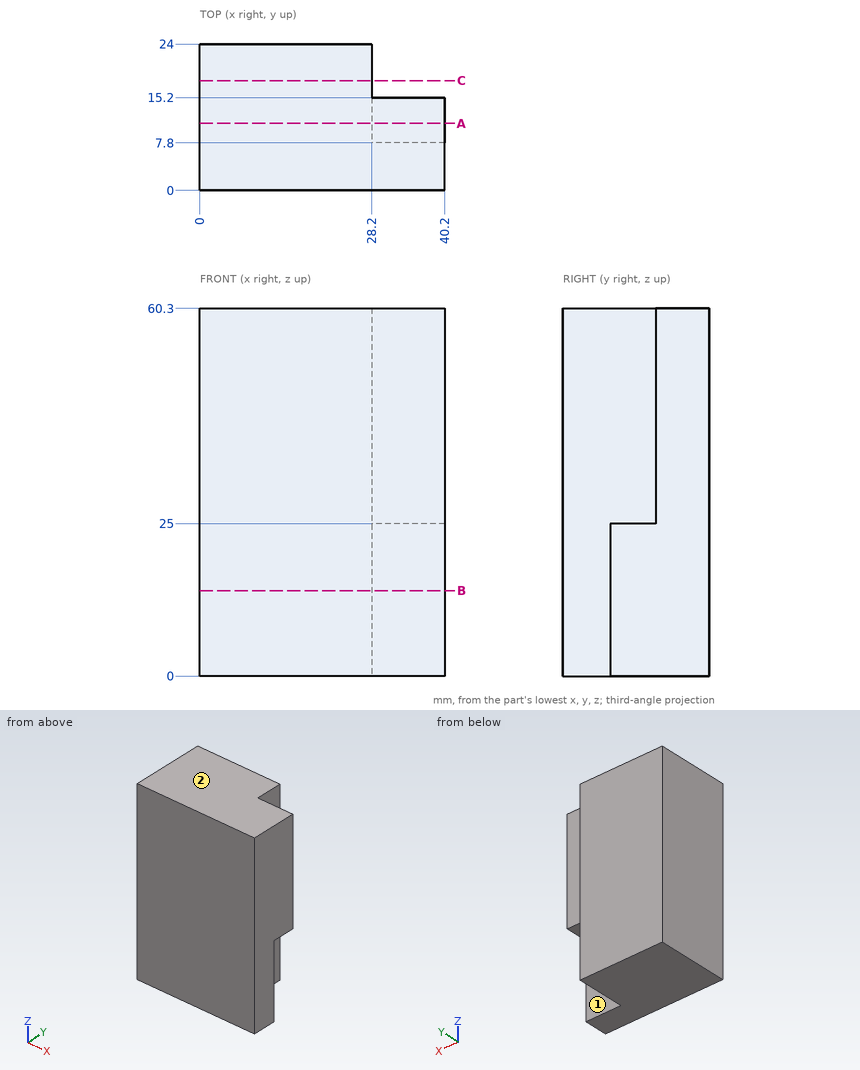
Drawing for the job (mm, zero at the part's lowest x, y, z). A direction names the side the tool comes from. Round coordinates to 2 decimals unless told otherwise and drop trailing zeros. Write each loop counter-clockwise with the first axis right and the second up, starting at its lowest first coordinate (ties: lowest second). Pieces come first, ordered by that corner, then holes.
Item 1: Band-saw the part on C-C on y = 18. Write the cut outline in (x, z).
Filled in:
outline: (0, 0) - (28.2, 0) - (28.2, 60.3) - (0, 60.3) - close
Item 2: Band-saw the part on A-A on y = 11. Write the cut outline in (x, z).
Filled in:
outline: (0, 0) - (28.2, 0) - (28.2, 25) - (40.2, 25) - (40.2, 60.3) - (0, 60.3) - close
Item 3: Drop flat-ended pins along their axis: pin 1 Ø2 at (x, y) = (34.5, 12.5) entering from -Z; pin 2 Ø2 at (y, z) = (18.5, 24.5) entering from +X; pin 3 Ø13 at (x, z) = (36, 14) entering from +Y. Give the stop position or say it passes through.
Filled in:
pin 1: stops at z = 25
pin 2: stops at x = 28.2
pin 3: stops at y = 7.8
Item 4: Drill centre lines: L1, parallel to Y at x = 37, z = 30.5; L2, parallel to X at y = 11.25, z = 13; L3, parallel to Y at x = 34.5, z = 6. Where is each one in solid material? Low to high.
Filled in:
L1: y = 0 to 15.2
L2: x = 0 to 28.2
L3: y = 0 to 7.8
Item 5: Band-saw the part on B-B on z = 14. Write the cut outline in (x, y), then the cut area to 3 significant figures.
Filled in:
outline: (0, 0) - (40.2, 0) - (40.2, 7.8) - (28.2, 7.8) - (28.2, 24) - (0, 24) - close
area: 770 mm2
Item 6: Tool access for the marked faces 1 and 2: list every direction of +Z, -Z, +X, -X, +Y, -Y with a clear straight run to the whole face (end or side of a thin tool).
Filled in:
face 1: -Z, +X, +Y
face 2: +Z, +X, -X, +Y, -Y
